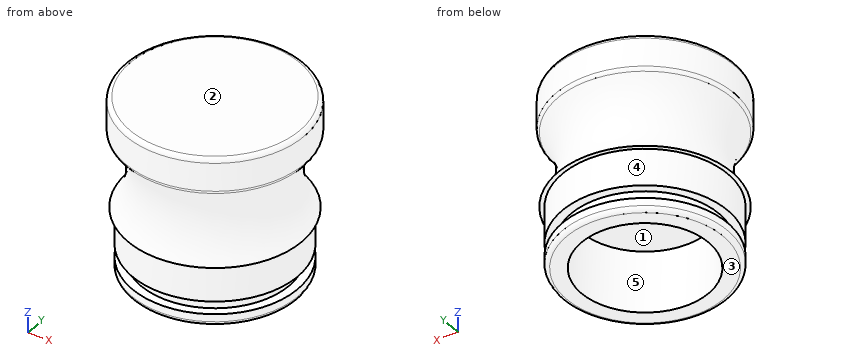
from build123d import *


# Not quite as in the source:
# - a fillet or chamfer that OpenCascade refuses, or shapes differently, is made with other operations: its cross-section is extruded or revolved along the edge and cut away or added


with BuildPart() as f1:
    # F0 (on Right) → F1 (revolve)
    with BuildSketch(Plane.YZ):
        with BuildLine():
            Line((7.5, 0), (7.5, -7.24))
            Line((7.5, -7.24), (9.75, -7.24))
            Line((9.75, -7.24), (9.75, -5.84))
            Line((9.75, -5.84), (8.75, -5.84))
            Line((8.75, -5.84), (8.75, -4.34))
            Line((8.75, -4.34), (9.75, -4.34))
            Line((9.75, -4.34), (9.75, 0))
            Line((9.75, 0), (10.25, 0))
            ThreePointArc((10.25, 0), (8.5974540278, 4.43), (10.25, 8.86))
            Line((10.25, 8.86), (10.5, 8.86))
            Line((10.5, 8.86), (10.5, 13.11))
            Line((10.5, 13.11), (0, 13.11))
            Line((0, 13.11), (0, 8.86))
            Line((0, 8.86), (0, 0))
            Line((0, 0), (7.5, 0))
        make_face()
    revolve(axis=Axis((0, 0, 4.43), (0, 0, 1)))

    # F2: fillet of radius 0.5 on 3 edges, made by hand

    # F2_s1 → F2_t2 (revolve, cut)
    with BuildSketch(Plane.YZ):
        with BuildLine():
            ThreePointArc((10.25, 8.86), (10.4330127019, 9.0430127019), (10.5, 9.2930127019))
            Line((10.5, 9.2930127019), (10.5, 8.86))
            Line((10.5, 8.86), (10.25, 8.86))
        make_face()
    revolve(axis=Axis((0, 0, 8.86), (0, 0, 1)), mode=Mode.SUBTRACT)

    # F2_s3 → F2_t4 (revolve, cut)
    with BuildSketch(Plane.YZ):
        with BuildLine():
            ThreePointArc((9.25, -7.24), (9.6035533906, -7.0935533906), (9.75, -6.74))
            Line((9.75, -6.74), (9.75, -7.24))
            Line((9.75, -7.24), (9.25, -7.24))
        make_face()
    revolve(axis=Axis((0, 0, -7.24), (0, 0, 1)), mode=Mode.SUBTRACT)

    # F2_s5 → F2_t6 (revolve, cut)
    with BuildSketch(Plane.YZ):
        with BuildLine():
            ThreePointArc((10.5, 12.61), (10.3535533906, 12.9635533906), (10, 13.11))
            Line((10, 13.11), (10.5, 13.11))
            Line((10.5, 13.11), (10.5, 12.61))
        make_face()
    revolve(axis=Axis((0, 0, 13.11), (0, 0, 1)), mode=Mode.SUBTRACT)


solid = f1.part
The model under review builds one solid part; all positions refer to its coordinate system, in mm. Face numbers are marked on the shaded views. A direction names the side the tool comes from. Round coordinates to 2 decimals unless told otherwise and drop trailing zeros. Order: outer loops, then holes, each group sorted by start corner. A loop starts at its lowest first (then second) coordinate and runs counter-clockwise, first axis right, second up. Notation, with made-up numbers: (10, 56) -> (68, 56) arc R30 ccw to (68, 80) -> close; hole circle Ø6 at (60.25, 25). An arc over 180 degrees is marked (long way). Write item = value, one per line. Start each with the question number.
Item 1: Consider section D-D on z = 2. Write out the cut boundary in (x, y).
Item 2: For the marked faces 1 and 2, list the 3-axis set-ups (+Z, -Z, +X, -X, +Y, -Y) from which the entire face can be reached by the end or side of a thin tool; tool diameter is ignored.
Item 3: For line 1 along X through (y, z) = (0, -5); line 2 along Y through (x, z) = (0, -2.5), list the stretches that pass through material, from the lowest coordinate up.
Item 4: Consider section C-C on z = 11.5. Write out the cut boundary in (x, y), plus the area to 3 significant figures.
Item 5: Consider section A-A on x = 0. Write out the cut boundary in (y, z).
Item 6: Clearance check with flat-ended pins moving along their axes: pin 1 Ø10 at (y, z) = (-7, -5) entering from +X; pin 2 Ø1.5 at (y, z) = (-1, 7) entering from +X; pin 3 Ø4 at (y, z) = (6, 7.5) entering from +X; pin 4 Ø6 at (x, y) = (2.5, 5) entering from -Z. State where each tip first meets the part, or that it passes through.
Item 7: Mouldability with a two-part tool opening along X and no side actions: class the marked faces 3, 4 and 5 as released by +X, released by -X, zero draft, split by the parting line, or undercut.
Conclusion:
q1.outline = circle Ø18.1 at (0, 0)
q2.face_1 = -Z
q2.face_2 = +Z, +X, -X, +Y, -Y
q3.line_1 = -8.75 to -7.5, 7.5 to 8.75
q3.line_2 = -9.75 to -7.5, 7.5 to 9.75
q4.outline = circle Ø21 at (0, 0)
q4.area = 346 mm2
q5.outline = (-10.5, 9.29) arc R0.5 ccw to (-10.25, 8.86) arc R6.76 cw to (-10.25, 0) -> (-9.75, 0) -> (-9.75, -4.34) -> (-8.75, -4.34) -> (-8.75, -5.84) -> (-9.75, -5.84) -> (-9.75, -6.74) arc R0.5 ccw to (-9.25, -7.24) -> (-7.5, -7.24) -> (-7.5, 0) -> (7.5, 0) -> (7.5, -7.24) -> (9.25, -7.24) arc R0.5 ccw to (9.75, -6.74) -> (9.75, -5.84) -> (8.75, -5.84) -> (8.75, -4.34) -> (9.75, -4.34) -> (9.75, 0) -> (10.25, 0) arc R6.76 cw to (10.25, 8.86) arc R0.5 ccw to (10.5, 9.29) -> (10.5, 12.61) arc R0.5 ccw to (10, 13.11) -> (-10, 13.11) arc R0.5 ccw to (-10.5, 12.61) -> close
q6.pin_1 = 9.53
q6.pin_2 = 9.42
q6.pin_3 = 9.3
q6.pin_4 = -7.24
q7.face_3 = zero draft
q7.face_4 = split by the parting line
q7.face_5 = undercut
